For this review, take the finished solid that the model builds, in its own axes (mm). A direction names the side the tool comes from. Give positions to 0.01 mm unless a question says otherwise; leave off trailing zeros. Order: outer loops, then holes, each group sorted by start corner. A loop starts at its lowest first (then second) coordinate and runs counter-clockwise, first axis right, second up. Notation, with made-up numbers: (45.25, 36.25) - (69.25, 36.25) arc R26 cw to (69.25, 55.25) - close; hole circle Ø1 at (5.25, -9). An arc over 180 degrees is marked (long way). Use a Markdown table: item, result. Add a question column.
1) We need section C-C on y = 1.25. Write out the cut boundary in (x, z).
2) Machinability: for faces 4 (the face through (2, 4, 50)), 5 (the face through (0, 0, 16)), 6 (the face through (0, 0, 18)), which of the approach directions +Z, -Z, +X, -X, +Y, -Y give a long, thin tool a straight path to every point of the face, cutting with its end or side? Answer none if there is none.
3) Clearance check with flat-ended pins moving along their axes: P1, Ø2, axis at x = -1.5, z = 38, coming from the -Y side; P2, Ø0.8, axis at y = -4.5, z = 31.5, coming from the -X side; P3, Ø3, axis at x = 1.5, y = -1.5, coming from the -Z side. State where each tip first meets the part, or that it passes through.
4) We need section D-D on x = -2. Write out the cut boundary in (y, z).
5) We need section A-A on x = 1. Write out the cut boundary in (y, z).
6) We need section B-B on z = -2. Write out the cut boundary in (x, y), then the cut area to 3 significant figures.
7) Wall thickness on L1, parallel to Z at x = 1, y = -3.75; L2, parallel to X at y = 2.5, z = 30; L3, parallel to Y at x = -1.5, z = 19.5: over which ranges is each line inside the solid? List them lowest first.
8) Mouldability with a two-part tool opening along X and no side actions: class faces 1 (the face through (2, 4, -25)), 2 (the face through (0, 0, 10)), 3 (the face through (0, 0, 12)) as released by +X, released by -X, zero draft, split by the parting line, or undercut.
```python
from build123d import *

# Parameters (mm, degrees)
F1_DEPTH = 50
F2_START = 16
F2_DEPTH = 2
F3_START = 10
F3_DEPTH = 2
F4_DEPTH = 25


with BuildPart() as f1:
    # F0 (on Top) → F1 (new body)
    with BuildSketch(Plane.XY):
        with BuildLine():
            ThreePointArc((-3.7313016861, -1.4427016245), (-0.7338010135, 3.9326246099), (4.0005, 0))
            ThreePointArc((4.0005, 0), (2.8287806781, -2.8287806781), (0, -4.0005))
            Line((0, -4.0005), (0, -5.0038))
            ThreePointArc((0, -5.0038), (3.5382209117, -3.5382209117), (5.0038, 0))
            ThreePointArc((5.0038, 0), (-0.9216629242, 4.9181858336), (-4.6642730222, -1.8117868569))
            Line((-4.6642730222, -1.8117868569), (-3.7313016861, -1.4427016245))
        make_face()
    extrude(amount=F1_DEPTH)

    # F0 (on Top) → F2 (join)
    with BuildSketch(Plane.XY.offset(F2_START)):
        with BuildLine():
            ThreePointArc((0, -4.0005), (2.8287806781, -2.8287806781), (4.0005, 0))
            ThreePointArc((4.0005, 0), (-0.7338010135, 3.9326246099), (-3.7313016861, -1.4427016245))
            ThreePointArc((-3.7313016861, -1.4427016245), (-2.2619098569, -3.2996612022), (0, -4.0005))
        make_face()
    extrude(amount=F2_DEPTH)

    # F0 (on Top) → F3 (join)
    with BuildSketch(Plane.XY.offset(F3_START)):
        with BuildLine():
            ThreePointArc((0, -4.0005), (2.8287806781, -2.8287806781), (4.0005, 0))
            ThreePointArc((4.0005, 0), (-0.7338010135, 3.9326246099), (-3.7313016861, -1.4427016245))
            ThreePointArc((-3.7313016861, -1.4427016245), (-2.2619098569, -3.2996612022), (0, -4.0005))
        make_face()
    extrude(amount=F3_DEPTH)

    # F0 (on Top) → F4 (join)
    with BuildSketch(Plane.XY):
        with BuildLine():
            ThreePointArc((-3.7313016861, -1.4427016245), (-0.7338010135, 3.9326246099), (4.0005, 0))
            ThreePointArc((4.0005, 0), (2.8287806781, -2.8287806781), (0, -4.0005))
            Line((0, -4.0005), (0, -5.0038))
            ThreePointArc((0, -5.0038), (3.5382209117, -3.5382209117), (5.0038, 0))
            ThreePointArc((5.0038, 0), (-0.9216629242, 4.9181858336), (-4.6642730222, -1.8117868569))
            Line((-4.6642730222, -1.8117868569), (-3.7313016861, -1.4427016245))
        make_face()
    extrude(amount=-F4_DEPTH)


solid = f1.part
```
Checked values:
| question | item | result |
|---|---|---|
| 1 | outline | (-4.85, -25) - (-3.8, -25) - (-3.8, 10) - (3.8, 10) - (3.8, -25) - (4.85, -25) - (4.85, 50) - (3.8, 50) - (3.8, 18) - (-3.8, 18) - (-3.8, 50) - (-4.85, 50) - close; hole (-3.8, 12) - (3.8, 12) - (3.8, 16) - (-3.8, 16) - close |
| 2 | face 4 | +Z, +X, -X, +Y, -Y |
| 2 | face 5 | none |
| 2 | face 6 | +Z |
| 3 | P1 | y = 3.12 |
| 3 | P2 | x = 0 |
| 3 | P3 | z = 10 |
| 4 | outline | (-3.46, 10) - (3.46, 10) - (3.46, -25) - (4.59, -25) - (4.59, 50) - (3.46, 50) - (3.46, 18) - (-3.46, 18) - (-3.46, 16) - (3.46, 16) - (3.46, 12) - (-3.46, 12) - close |
| 5 | outline | (-4.9, -25) - (-3.87, -25) - (-3.87, 10) - (3.87, 10) - (3.87, -25) - (4.9, -25) - (4.9, 50) - (3.87, 50) - (3.87, 18) - (-3.87, 18) - (-3.87, 50) - (-4.9, 50) - close; hole (-3.87, 12) - (3.87, 12) - (3.87, 16) - (-3.87, 16) - close |
| 6 | outline | (-4.66, -1.81) - (-3.73, -1.44) arc R4 cw (long way) to (0, -4) - (0, -5) arc R5 ccw (long way) to start |
| 6 | area | 23.0 mm² |
| 7 | L1 | 10 to 12, 16 to 18 |
| 7 | L2 | -4.33 to -3.12, 3.12 to 4.33 |
| 7 | L3 | 3.71 to 4.77 |
| 8 | face 1 | zero draft |
| 8 | face 2 | undercut |
| 8 | face 3 | undercut |
